Geometry: final body of the model. Coordinates: model frame, mm. Round coordinates to 2 decimals unless told otherwise and drop trailing zeros. Write each loop counter-clockwise with the first axis right and the second up, starting at its lowest first coordinate (ties: lowest second). Pieces come first, ordered by that corner, then holes. Notation, with made-up numbers: M 18.25,10 L 22.25,10 A35 cw 22.25,44 Z; hole C 27,32 d4. An arc over 180 degrees is marked long. Use one line per item in the form item = value. Start each with the question number.
Item 1: Ray query, probe 1 along Y at (x, z) = (1.5, 1); probe 2 along X at (y, z) = (97.5, 6); probe 3 along Y at (x, z) = (21, 6). Return the intervals inside material, ascending.
Item 2: Section query A-A (x = 8). Return loops of the section in (y, z), and give its area (3 significant figures).
Item 3: Pin query (flat end, axial travel): pin 1 Ø3 at (x, z) = (148, 2) entering from -Y; pin 2 Ø2 at (x, z) = (103, 3) entering from +Y; pin 3 Ø2 at (y, z) = (53, 3) entering from -X. Return the tip coordinate at first contact, or that it passes through.
Item 4: Section query B-B (y = 74). Return loops of the section in (x, z).
Item 5: Section query C-C (x = 118.5). Return loops of the section in (y, z), and give its area (3 significant figures).
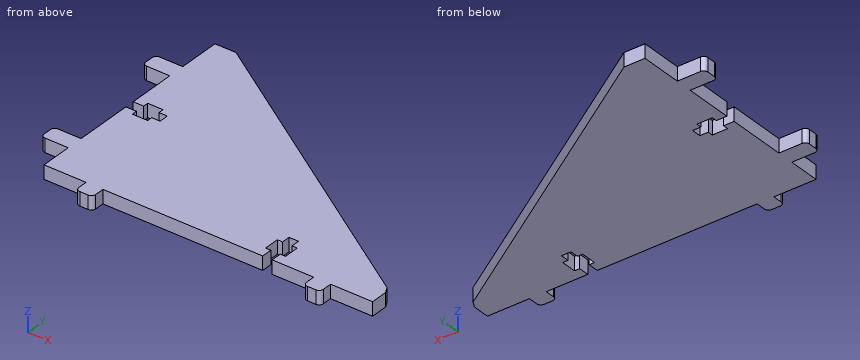
Autodesk Inventor part; units mm, degrees
ref_plane "YZ Plane" through (0, 0, 0) normal (1, 0, 0) x (0, 1, 0)
ref_plane "XZ Plane" through (0, 0, 0) normal (0, 1, 0) x (-1, 0, 0)
ref_plane "XY Plane" through (0, 0, 0) normal (0, 0, 1) x (1, 0, 0)
sketch "Sketch1" plane through (0, 0, 0) normal (0, 0, 1) x (1, 0, 0)
  line L0 (0, 106) -> (0, 0)
  line L1 (0, 0) -> (156.25, 0)
  line L2 (156.25, 0) -> (156.25, 10)
  line L3 (156.25, 10) -> (10, 106)
  line L4 (10, 106) -> (0, 106)
  dimension "d0" = 156.25
  dimension "d1" = 106
  dimension "d2" = 10
  dimension "d3" = 10
extrude "Extrusion1" add sketch "Sketch1" along normal blind 6.5
sketch "Sketch2" plane through (0, 0, 6.5) normal (0, 0, 1) x (1, 0, 0)
  line L0 (0, 106) -> (0, 0)
  line L1 (0, 0) -> (156.25, 0)
  line L2 (156.25, 0) -> (156.25, 10)
  line L3 (16.3, 55.25) -> (16.3, 50.75)
  line L4 (0, 50.75) -> (0, 55.25)
  line L5 (5, 57.75) -> (12.3, 57.75)
  line L6 (12.3, 48.25) -> (5, 48.25)
  line L7 (0, 55.25) -> (5, 55.25)
  line L8 (12.3, 55.25) -> (16.3, 55.25)
  line L9 (16.3, 50.75) -> (12.3, 50.75)
  line L10 (5, 50.75) -> (0, 50.75)
  line L11 (5, 48.25) -> (5, 50.75)
  line L12 (5, 55.25) -> (5, 57.75)
  line L13 (12.3, 57.75) -> (12.3, 55.25)
  line L14 (12.3, 50.75) -> (12.3, 48.25)
  line L15 (104, 16.3) -> (108.5, 16.3)
  line L16 (108.5, 0) -> (104, 0)
  line L17 (111, 12.3) -> (111, 5)
  line L18 (101.5, 5) -> (101.5, 12.3)
  line L19 (101.5, 12.3) -> (104, 12.3)
  line L20 (108.5, 12.3) -> (111, 12.3)
  line L21 (111, 5) -> (108.5, 5)
  line L22 (104, 5) -> (101.5, 5)
  line L23 (104, 0) -> (104, 5)
  line L24 (104, 12.3) -> (104, 16.3)
  line L25 (108.5, 16.3) -> (108.5, 12.3)
  line L26 (108.5, 5) -> (108.5, 0)
  point P0 (16.3, 53)
  point P1 (0, 53)
  point P2 (106.25, 16.3)
  dimension "d6" = 4.5
  dimension "d7" = 2.5
  dimension "d8" = 2.5
  dimension "d9" = 5
  dimension "d10" = 7.3
  dimension "d11" = 4
  dimension "d12" = 4.5
  dimension "d13" = 5
  dimension "d14" = 7.3
  dimension "d15" = 4
  dimension "d16" = 2.5
  dimension "d17" = 2.5
  dimension "d18" = 50
extrude "Extrusion2" cut sketch "Sketch2" against normal through all
sketch "Sketch3" plane through (0, 0, 6.5) normal (0, 0, 1) x (1, 0, 0)
  line L0 (0, 50.75) -> (0, 0)
  line L1 (0, 0) -> (104, 0)
  line L2 (108.5, 0) -> (156.25, 0)
  line L3 (10, 106) -> (0, 106)
  line L4 (0, 106) -> (0, 55.25)
  line L5 (0, 86) -> (-11, 86)
  line L6 (-13, 84) -> (-13, 80)
  line L7 (-11, 78) -> (0, 78)
  line L8 (0, 78) -> (0, 86)
  line L9 (0, 23) -> (-11, 23)
  line L10 (-13, 21) -> (-13, 17)
  line L11 (-11, 15) -> (0, 15)
  line L12 (0, 15) -> (0, 23)
  line L13 (20, 0) -> (28, 0)
  line L14 (28, 0) -> (28, -4.5)
  line L15 (26, -6.5) -> (22, -6.5)
  line L16 (20, -4.5) -> (20, 0)
  line L17 (128.25, 0) -> (136.25, 0)
  line L18 (136.25, 0) -> (136.25, -4.5)
  line L19 (134.25, -6.5) -> (130.25, -6.5)
  line L20 (128.25, -4.5) -> (128.25, 0)
  arc A0 (-11, 86) -> (-13, 84) centre (-11, 84) ccw
  arc A1 (-13, 80) -> (-11, 78) centre (-11, 80) ccw
  arc A2 (-11, 23) -> (-13, 21) centre (-11, 21) ccw
  arc A3 (-13, 17) -> (-11, 15) centre (-11, 17) ccw
  arc A4 (20, -4.5) -> (22, -6.5) centre (22, -4.5) ccw
  arc A5 (26, -6.5) -> (28, -4.5) centre (26, -4.5) ccw
  arc A6 (128.25, -4.5) -> (130.25, -6.5) centre (130.25, -4.5) ccw
  arc A7 (134.25, -6.5) -> (136.25, -4.5) centre (134.25, -4.5) ccw
  dimension "d21" = 2
  dimension "d22" = 8
  dimension "d23" = 8
  dimension "d24" = 8
  dimension "d25" = 8
  dimension "d26" = 13
  dimension "d27" = 6.5
  dimension "d28" = 15
  dimension "d29" = 20
  dimension "d30" = 20
  dimension "d31" = 20
extrude "Extrusion3" add sketch "Sketch3" against normal blind 6.5
chamfer "Chamfer1" distance 2 angle 45 1 edges at (156.25, 10, 3.25)
properties part number "wiring_brace" material "Plywood, Finish"
Working result:
q1.probe_1 = 0 to 50.75, 55.25 to 106
q1.probe_2 = 0 to 22.95
q1.probe_3 = -6.23 to 98.78
q2.outline = M 0,0 L 48.25,0 L 48.25,6.5 L 0,6.5 Z; M 57.75,0 L 106,0 L 106,6.5 L 57.75,6.5 Z
q2.area = 627 mm²
q3.pin_1 = 0
q3.pin_2 = 45.61
q3.pin_3 = 16.3
q4.outline = M 0,0 L 58.75,0 L 58.75,6.5 L 0,6.5 Z
q5.outline = M 0,0 L 34.78,0 L 34.78,6.5 L 0,6.5 Z
q5.area = 226 mm²
